Read the model definition and answer for the solid it produces. Units are mm, in the model's axes. Coordinates: 2 decimals unless noted, no trailing zeros. Loops run counter-clockwise (first coordinate to the right, second up) from the corner with the lowest first, then second, coordinate; pieces in that order, holes last. Notation, with made-up numbers: (41.5, 62) - (78.5, 62) arc R21 cw to (78.5, 89) - close; hole circle Ø1 at (-6.75, 62). An arc over 180 degrees is marked (long way). Use one line per item in the form item = value.
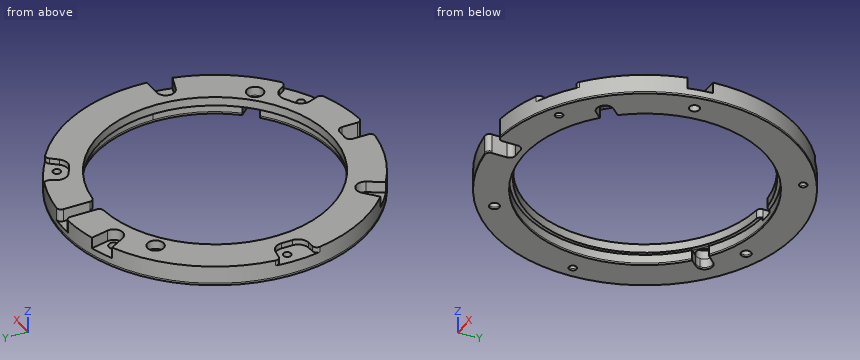
from build123d import *
from build123d.topology import SkipClean

# Parameters (mm, degrees)
CUT_EXTRUDE_1_DEPTH              = 3
SKETCH_3_R                       = 0.425
CUT_EXTRUDE_2_DEPTH              = 10
CUT_EXTRUDE_3_DEPTH              = 0.61
FILLET_1_R                       = 0.5
PATTERN_CIRCULAR_1_COUNT         = 3
FILLET_1_OF_PATTERN_CIRCULAR_1_R = 0.5
SKETCH_5_W                       = 1.5
SKETCH_5_H                       = 10.413141387
CUT_EXTRUDE_4_DEPTH              = 1.4
FILLET_2_R                       = 0.6
SKETCH_22_R                      = 0.9
CUT_EXTRUDE_14_DEPTH             = 24.697731959
FILLET_3_R                       = 0.5
SKETCH_14_R                      = 0.55
CUT_EXTRUDE_9_DEPTH              = 24.697731959
CUT_EXTRUDE_10_DEPTH             = 1.23
SKETCH_23_R                      = 13.2
SKETCH_23_R_2                    = 0.425
SKETCH_23_R_3                    = 0.9
SKETCH_23_R_4                    = 0.55
EXTRUDE_1_DEPTH                  = 0.23
CUT_EXTRUDE_15_DEPTH             = 1.2


with BuildPart() as part:
    # Эскиз1 → Повернуть1 (revolve)
    with BuildSketch(Plane(origin=(0, 0, 0), x_dir=(1, 0, 0), z_dir=(0, 1, 0)), mode=Mode.PRIVATE) as revolve_1_sk:
        Polygon((-16.7, 0), (-12.825, 0), (-12.825, 0.98), (-13.2, 0.98), (-13.2, 1.95), (-16.7, 1.95), align=None)
    revolve(revolve_1_sk.sketch.rotate(Axis((0, 0, 0), (0, 0, -1)), 180), axis=Axis((0, 0, 0), (0, 0, -1)))

    # Эскиз2 → Вырез-Вытянуть1 (cut)
    with BuildSketch(Plane(origin=(0, 0, -1.95), x_dir=(-1, 0, 0), z_dir=(0, 0, -1))):
        with BuildLine():
            Line((1.15, -16.660357139), (1.15, -13.86))
            Line((1.15, -13.86), (-1.15, -13.86))
            Line((-1.15, -13.86), (-1.15, -16.660357139))
            ThreePointArc((-1.15, -16.660357139), (0, -16.850858655), (1.15, -16.660357139))
        make_face()
    extrude(amount=-CUT_EXTRUDE_1_DEPTH, mode=Mode.SUBTRACT)

    # Эскиз3 → Вырез-Вытянуть2 (cut)
    with BuildSketch(Plane.XY):
        with Locations((-15.37, 0)):
            Circle(SKETCH_3_R)
    cut_extrude_2 = extrude(amount=-CUT_EXTRUDE_2_DEPTH, mode=Mode.SUBTRACT)

    # Эскиз4 → Вырез-Вытянуть3 (cut)
    with BuildSketch(Plane.XY):
        with BuildLine():
            Line((-15.183288241, 1.185390734), (-17.344587168, 1.525820031))
            Line((-17.344587168, 1.525820031), (-17.293113612, -0.525872079))
            Line((-17.293113612, -0.525872079), (-16.759364893, -2.507589098))
            Line((-16.759364893, -2.507589098), (-15.275238911, -2.391362418))
            ThreePointArc((-15.275238911, -2.391362418), (-14.487532806, -2.009361072), (-14.168928398, -1.193948803))
            Line((-14.168928398, -1.193948803), (-14.170000491, 0.001081813))
            ThreePointArc((-14.170000491, 0.001081813), (-14.458194682, 0.780140539), (-15.183288241, 1.185390734))
        make_face()
    cut_extrude_3 = extrude(amount=-CUT_EXTRUDE_3_DEPTH, mode=Mode.SUBTRACT)

    # Скругление1
    fillet_1_edges = [part.edges().sort_by_distance(p)[0] for p in [
        (-16.513575068, -2.488340506, -0.305),
        (-16.639959355, 1.414833093, -0.305),
    ]]
    fillet(fillet_1_edges, radius=FILLET_1_R)

    # Круговой массив1: Вырез-Вытянуть2, Вырез-Вытянуть3 ×3 about axis
    pattern_circular_1_axis = Axis((0, 0, 0), (0, 0, 1))
    add([cut_extrude_2.rotate(pattern_circular_1_axis, i * 360 / PATTERN_CIRCULAR_1_COUNT) for i in range(1, PATTERN_CIRCULAR_1_COUNT)], mode=Mode.SUBTRACT)
    add([cut_extrude_3.rotate(pattern_circular_1_axis, i * 360 / PATTERN_CIRCULAR_1_COUNT) for i in range(1, PATTERN_CIRCULAR_1_COUNT)], mode=Mode.SUBTRACT)

    # Скругление1 of Круговой массив1
    fillet_1_of_pattern_circular_1_edges = [part.edges().sort_by_distance(p)[0] for p in [
        (10.411753626, -13.057005263, -0.305),
        (7.094698277, -15.118044065, -0.305),
        (6.101821442, 15.545345769, -0.305),
        (9.545261078, 13.703210973, -0.305),
    ]]
    fillet(fillet_1_of_pattern_circular_1_edges, radius=FILLET_1_OF_PATTERN_CIRCULAR_1_R)

    # Эскиз5 → Вырез-Вытянуть4 (cut)
    with BuildSketch(Plane.XY):
        with Locations((0, 14.598970831)):
            Rectangle(SKETCH_5_W, SKETCH_5_H)
    extrude(amount=-CUT_EXTRUDE_4_DEPTH, mode=Mode.SUBTRACT)

    # Скругление2
    fillet_2_edges = [part.edges().sort_by_distance(p)[0] for p in [
        (1.15, -13.86, -0.975),
        (-1.15, -13.86, -0.975),
    ]]
    fillet(fillet_2_edges, radius=FILLET_2_R)

    # Эскиз22 → Вырез-Вытянуть14 (cut, through all)
    with BuildSketch(Plane(origin=(0, 0, -1.95), x_dir=(-1, 0, 0), z_dir=(0, 0, -1))):
        with Locations((-10.425450224, -9.714550304)):
            Circle(SKETCH_22_R)
        with Locations((8.963643503, 11.077707125)):
            Circle(SKETCH_22_R)
    extrude(amount=-CUT_EXTRUDE_14_DEPTH, mode=Mode.SUBTRACT)

    # Скругление3
    # the kernel refuses this fillet: 0.5 mm, written as the material it takes off along each edge
    with BuildSketch(Plane(origin=(-0.75, 12.803051394, 1.157971634), x_dir=(0, 1, 0), z_dir=(0, 0, -1))) as fillet_3_piece_1_section:
        with BuildLine():
            CenterArc((0.463188653, -0.5), FILLET_3_R, 90, 84.617246865)
            ThreePointArc((-0.03460647, -0.453095685), (-0.015296317, -0.226701126), (0, 0))
            Line((0, 0), (0.463188653, 0))
        make_face()
    fillet_3_piece_1 = extrude(amount=3.295943267, mode=Mode.PRIVATE)
    fillet_3_piece_1 = split(fillet_3_piece_1, bisect_by=Plane(origin=(-0.752336833, 13.200365704, -1.4), z_dir=(0, 0, 1)), keep=Keep.TOP, mode=Mode.PRIVATE)
    add(fillet_3_piece_1, mode=Mode.SUBTRACT)
    with BuildSketch(Plane(origin=(0.75, 12.803051394, 1.157971634), x_dir=(0.9970959124373047, -0.07615603325291273, 0), z_dir=(0, 0, -1))) as fillet_3_piece_2_section:
        with BuildLine():
            CenterArc((0.463273346, -0.49992153), FILLET_3_R, 91.015105015, 84.617246865)
            Line((-0.03527461, -0.461843513), (0, 0))
            ThreePointArc((0, 0), (0.227207673, -0.002012763), (0.454415347, 0))
        make_face()
    fillet_3_piece_2 = extrude(amount=3.295943267, mode=Mode.PRIVATE)
    fillet_3_piece_2 = split(fillet_3_piece_2, bisect_by=Plane(origin=(0.850744081, 12.897606018, -1.4), z_dir=(0, 0, 1)), keep=Keep.TOP, mode=Mode.PRIVATE)
    add(fillet_3_piece_2, mode=Mode.SUBTRACT)
    with BuildSketch(Plane(origin=(0.75, 16.683150182, -1.4), x_dir=(0.9981351186761567, -0.061043303198095235, 0), z_dir=(0, 0, 1))) as fillet_3_piece_3:
        with BuildLine():
            CenterArc((0.531508869, -0.499934747), FILLET_3_R, 89.074330097, 94.425369323)
            Line((0.03244131, -0.530456399), (0, 0))
            ThreePointArc((0, 0), (0.269793256, 0.002179436), (0.539586512, 0))
        make_face()
    extrude(amount=2.748966279, mode=Mode.SUBTRACT)
    with BuildSketch(Plane(origin=(-0.75, 16.683150182, -1.4), x_dir=(-0.9981351186761567, -0.06104330319809576, 0), z_dir=(0, 0, 1))) as fillet_3_piece_4:
        with BuildLine():
            CenterArc((0.531508869, 0.499934747), FILLET_3_R, 176.500300581, 94.425369323)
            Line((0.03244131, 0.530456399), (0, 0))
            ThreePointArc((0, 0), (0.269793256, -0.002179436), (0.539586512, 0))
        make_face()
    extrude(amount=2.748966279, mode=Mode.SUBTRACT)
    with BuildSketch(Plane(origin=(-1.15, -16.660357139, -3.33236123), x_dir=(-0.9963494237820577, 0.08536876319334569, 0), z_dir=(0, 0, 1))) as fillet_3_piece_5:
        with BuildLine():
            CenterArc((0.54466688, -0.499931476), FILLET_3_R, 89.051412184, 95.845818339)
            Line((0.046492168, -0.542615858), (0, 0))
            ThreePointArc((0, 0), (0.276472246, 0.002288687), (0.552944492, 0))
        make_face()
    extrude(amount=4.71472246, mode=Mode.SUBTRACT)
    with BuildSketch(Plane(origin=(1.15, -16.660357139, -3.33236123), x_dir=(0, 1, 0), z_dir=(0, 0, 1))) as fillet_3_piece_6:
        with BuildLine():
            CenterArc((0.544603976, -0.5), FILLET_3_R, 90, 95.845818339)
            ThreePointArc((0.047204187, -0.550925926), (0.021321762, -0.275658345), (0, 0))
            Line((0, 0), (0.544603976, 0))
        make_face()
    extrude(amount=4.71472246, mode=Mode.SUBTRACT)

    # Эскиз14 → Вырез-Вытянуть9 (cut, through all)
    with BuildSketch(Plane.XY):
        with Locations((-5.497143352, 13.848877751)):
            Circle(SKETCH_14_R)
        with Locations((-9.24490827, -11.685104667)):
            Circle(SKETCH_14_R)
        with Locations((14.742051622, -2.163773084)):
            Circle(SKETCH_14_R)
    extrude(amount=-CUT_EXTRUDE_9_DEPTH, mode=Mode.SUBTRACT)

    # Эскиз15 → Вырез-Вытянуть10 (cut)
    with BuildSketch(Plane.XY):
        with BuildLine():
            Line((-7.888402349, 15.883675138), (-5.15235159, 16.969717163))
            Line((-5.15235159, 16.969717163), (-4.519975471, 14.06134641))
            ThreePointArc((-4.519975471, 14.06134641), (-5.128207557, 12.919422868), (-6.354014422, 13.333346986))
            Line((-6.354014422, 13.333346986), (-7.888402349, 15.883675138))
        make_face()
        with BuildLine():
            Line((17.699867349, -1.110280739), (17.272381953, -4.022791215))
            Line((17.272381953, -4.022791215), (14.437470938, -3.116259623))
            ThreePointArc((14.437470938, -3.116259623), (13.752652185, -2.018553414), (14.724024418, -1.163935587))
            Line((14.724024418, -1.163935587), (17.699867349, -1.110280739))
        make_face()
        with BuildLine():
            Line((-9.811465, -14.773394399), (-12.120030363, -12.946925948))
            Line((-12.120030363, -12.946925948), (-9.917495467, -10.945086787))
            ThreePointArc((-9.917495467, -10.945086787), (-8.624444628, -10.900869454), (-8.370009996, -12.169411398))
            Line((-8.370009996, -12.169411398), (-9.811465, -14.773394399))
        make_face()
    extrude(amount=-CUT_EXTRUDE_10_DEPTH, mode=Mode.SUBTRACT)

    # Эскиз23 → Бобышка-Вытянуть1 (add)
    with SkipClean():  # the faces are left unmerged after this step: merging them gives an invalid solid
        with BuildSketch(Plane(origin=(0, 0, -1.95), x_dir=(-1, 0, 0), z_dir=(0, 0, -1))):
            with BuildLine():
                Line((1.15, -14.46), (1.15, -16.115753163))
                ThreePointArc((1.15, -16.115753163), (1.314935053, -16.486875085), (1.700925926, -16.613152952))
                ThreePointArc((1.700925926, -16.613152952), (0, 16.7), (-1.700925926, -16.613152952))
                ThreePointArc((-1.700925926, -16.613152952), (-1.314935053, -16.486875085), (-1.15, -16.115753163))
                Line((-1.15, -16.115753163), (-1.15, -14.46))
                ThreePointArc((-1.15, -14.46), (-0.974264069, -14.035735931), (-0.55, -13.86))
                Line((-0.55, -13.86), (0.55, -13.86))
                ThreePointArc((0.55, -13.86), (0.974264069, -14.035735931), (1.15, -14.46))
            make_face()
            with Locations(Location((0, 0, 0), (0, 0, 93.291137806))):
                Circle(SKETCH_23_R, mode=Mode.SUBTRACT)
            with Locations(Location((15.37, 0, 0), (0, 0, 180))):
                Circle(SKETCH_23_R_2, mode=Mode.SUBTRACT)
            with Locations(Location((-7.685, -13.310810456, 0), (0, 0, 180))):
                Circle(SKETCH_23_R_2, mode=Mode.SUBTRACT)
            with Locations(Location((-7.685, 13.310810456, 0), (0, 0, 180))):
                Circle(SKETCH_23_R_2, mode=Mode.SUBTRACT)
            with Locations((8.963643503, 11.077707125)):
                Circle(SKETCH_23_R_3, mode=Mode.SUBTRACT)
            with Locations((-10.425450224, -9.714550304)):
                Circle(SKETCH_23_R_3, mode=Mode.SUBTRACT)
            with Locations(Location((-14.742051622, -2.163773084, 0), (0, 0, 180))):
                Circle(SKETCH_23_R_4, mode=Mode.SUBTRACT)
            with Locations(Location((9.24490827, -11.685104667, 0), (0, 0, 180))):
                Circle(SKETCH_23_R_4, mode=Mode.SUBTRACT)
            with Locations(Location((5.497143352, 13.848877751, 0), (0, 0, 180))):
                Circle(SKETCH_23_R_4, mode=Mode.SUBTRACT)
        extrude(amount=EXTRUDE_1_DEPTH)

    # Эскиз24 → Вырез-Вытянуть15 (cut)
    with SkipClean():  # the faces are left unmerged after this step: merging them gives an invalid solid
        with BuildSketch(Plane(origin=(0, 0, -2.18), x_dir=(-1, 0, 0), z_dir=(0, 0, -1))):
            with BuildLine():
                Line((-9.767231893, -10.328348828), (9.621861835, 10.463908601))
                ThreePointArc((9.621861835, 10.463908601), (9.577442027, 11.735925456), (8.305425172, 11.691505649))
                Line((8.305425172, 11.691505649), (-11.083668556, -9.10075178))
                ThreePointArc((-11.083668556, -9.10075178), (-11.039248749, -10.372768636), (-9.767231893, -10.328348828))
            make_face()
        extrude(amount=-CUT_EXTRUDE_15_DEPTH, mode=Mode.SUBTRACT)


solid = part.part
Item 1: The part is cut by section A-A on x = 0. Give the vertices of the cut face in (y, z) (3 decimals), plus the area to 3 significant figures.
Results below:
outline = (-13.86, -2.18) - (-13.2, -2.18) - (-13.2, -0.98) - (-12.825, -0.98) - (-12.825, 0) - (-13.86, 0) - close; (13.2, -2.18) - (16.7, -2.18) - (16.7, -1.4) - (13.2, -1.4) - close
area = 4.54 mm²
Item 2: Each of these flat-tipped pins is pushed along its axis until it touches: P1, Ø0.8, axis at y = -15.5, z = -1, coming from the -X side; P2, Ø0.8, axis at x = 0, y = 14, coming from the +Z side; P3, Ø2, axis at x = -15.5, y = -1, coming from the +Z side; P4, Ø0.7, axis at x = 14.74, y = -2.16, coming from the +Z side. Where does it stop, or does it pass through?
Results below:
P1 = -7.13
P2 = -1.4
P3 = -0.61
P4 = through
Item 3: The part is cut by section B-B on y = 6.5. Give the vertices of the cut face in (x, z), plus the area to 3 significant figures.
Results below:
outline = (-15.38, -2.18) - (-11.49, -2.18) - (-11.49, -0.98) - (-11.06, -0.98) - (-11.06, 0) - (-15.38, 0) - close; (11.06, -0.98) - (11.49, -0.98) - (11.49, -2.18) - (15.38, -2.18) - (15.38, 0) - (11.06, 0) - close
area = 17.8 mm²
Item 4: The part is cut by section C-C on x = 4. Give the vertices of the cut face in (y, z), plus the area to 3 significant figures.
Results below:
outline = (-16.21, -2.18) - (-12.58, -2.18) - (-12.58, -0.98) - (-12.19, -0.98) - (-12.19, 0) - (-16.21, 0) - close; (12.19, -0.98) - (12.58, -0.98) - (12.58, -2.18) - (16.21, -2.18) - (16.21, 0) - (12.19, 0) - close
area = 16.6 mm²
Item 5: Find the intervals of material crossed by L1, parallel to X at y = 4.5, z = -0.25; L2, parallel to Y at x = -2.5, z = -0.3; L3, parallel to Y at x = -8.5, z = -1.7, in increasing order.
Results below:
L1 = -16.08 to -12.01, 12.01 to 16.08
L2 = -16.51 to -12.58, 12.58 to 16.51
L3 = -14.37 to -10.1, 11.85 to 14.37
